Can you work these out from the model? Positions are in its coordinate system, mm. Face numbers are marked on the shaded views. A direction names the side the tool comes from. Give positions to 0.01 mm unless a question says otherwise; leave off trailing zeros. Loops run counter-clockwise (first coordinate to the right, second up) from the corner with the lowest first, then second, coordinate; pieces in that order, holes last. Notation, with made-up numbers: (19, 50.25) -> (77, 50.25) arc R11 cw to (77, 68.25) -> close; hole circle Ø10 at (4, 67.5). An arc over 180 degrees is marked (long way). Return JSON: item names as keys, results as strings. Group by question number.
Q1. Suppose I cut it at A-A, the plane z = 52. Please give me the cut outline in (x, y), and give its area (3 significant figures).
Q2. I need wall thicknesses on line 1 along X through (y, z) = (4.5, 71.5); line 2 along Z through (x, y) = (110, 6); line 3 along Z through (x, y) = (199.51, -9.5). Which ranges of each line are inside material? Lowest first, please. Write a range as [from, to].
Q3. Suppose I cut it at C-C, the plane y = 15.5. Count the separate pieces of the cut face and the enclosed holes in it, and give its area (3 significant figures).
Q4. Which directions (+Z, -Z, +X, -X, +Y, -Y) give clear straight access to the entire face, cutting with the end or side of a thin tool? Please do the marked faces 5, 6 and 7.
Q5. Thinking about a two-plate mould opening in Z: for the marked faces 1, 2, 3 and 4, which applies, pulls with the +Z half, pulls with the -Z half, needs draft (parallel to the pull), parting line crosses it, or undercut?
Q6. Will these pins go through, and if not, where does the flat tip stop? pin 1 (2 mm diameter, centred on y = -9, z = 119, fed in from -X); pin 2 (5 mm diameter, centred on x = 99.5, y = 15.5, fed in from +Z); pin 3 (6 mm diameter, centred on x = 110.5, z = 111.5, fed in from -Y).
Q7. Suppose I cut it at B-B, the plane x = 156. Please give me the cut outline in (y, z).
```python
from build123d import *

# Parameters (mm, degrees)
PAD024_DEPTH    = 34.5
POCKET023_DEPTH = 31.5
SKETCH055_R     = 2.1
SKETCH055_R_2   = 2
POCKET024_DEPTH = 6.2
SKETCH057_R     = 3
SKETCH057_R_2   = 5
SKETCH057_R_3   = 3.5
PAD025_DEPTH    = 17.5
SKETCH058_R     = 2.55
SKETCH058_R_2   = 2.1
POCKET026_DEPTH = 6.2
FILLET001_R     = 3
SKETCH059_W     = 20
SKETCH059_H     = 10
POCKET027_DEPTH = 5
SKETCH060_W     = 20
SKETCH060_H     = 10
POCKET028_DEPTH = 5


with BuildPart() as part:
    # Sketch052 → Pad024 (new body)
    with BuildSketch(Plane.XZ):
        with BuildLine():
            ThreePointArc((-0.5, 13.5), (2.428932, 6.428932), (9.5, 3.5))
            Line((9.5, 3.5), (192.51, 3.5))
            ThreePointArc((192.51, 3.5), (199.581068, 6.428932), (202.51, 13.5))
            Line((202.51, 13.5), (202.51, 109.54))
            ThreePointArc((202.51, 109.54), (199.581068, 116.611068), (192.51, 119.54))
            Line((192.51, 119.54), (97.391395, 119.54))
            ThreePointArc((97.391395, 119.54), (96.36955, 119.672723), (95.415517, 120.062083))
            Line((95.415517, 120.062083), (67.291034, 136.040187))
            ThreePointArc((67.291034, 136.040187), (65.859984, 136.624227), (64.327218, 136.823311))
            Line((64.327218, 136.823311), (35.377399, 136.823311))
            ThreePointArc((35.377399, 136.823311), (30.31762, 135.448776), (26.64881, 131.703038))
            Line((26.64881, 131.703038), (2.447131, 88.412394))
            ThreePointArc((2.447131, 88.412394), (0.24888, 82.945607), (-0.5, 77.101188))
            Line((-0.5, 77.101188), (-0.5, 13.5))
        make_face()
    extrude(amount=PAD024_DEPTH)

    # Sketch054 (on Face16 of Pad024) → Pocket023 (cut)
    with BuildSketch(Plane.XZ.offset(34.5)):
        with BuildLine():
            ThreePointArc((5.5, 15.5), (8.428932, 8.428932), (15.5, 5.5))
            Line((15.5, 5.5), (186.51, 5.5))
            ThreePointArc((186.51, 5.5), (193.581068, 8.428932), (196.51, 15.5))
            Line((196.51, 15.5), (196.51, 107.54))
            ThreePointArc((196.51, 107.54), (193.581068, 114.611068), (186.51, 117.54))
            Line((186.51, 117.54), (96.852925, 117.54))
            ThreePointArc((96.852925, 117.54), (95.816521, 117.676599), (94.850903, 118.077066))
            Line((94.850903, 118.077066), (67.278075, 134.017712))
            ThreePointArc((67.278075, 134.017712), (65.829649, 134.618413), (64.275043, 134.823311))
            Line((64.275043, 134.823311), (41.153265, 134.823311))
            ThreePointArc((41.153265, 134.823311), (36.151908, 133.482781), (32.491444, 129.820596))
            Line((32.491444, 129.820596), (8.601898, 88.412711))
            ThreePointArc((8.601898, 88.412711), (6.288899, 82.824921), (5.5, 76.829005))
            Line((5.5, 76.829005), (5.5, 15.5))
        make_face()
    extrude(amount=-POCKET023_DEPTH, mode=Mode.SUBTRACT)

    # Sketch055 (on Face5 of Pocket023) → Pocket024 (cut)
    with BuildSketch(Plane.XZ.offset(34.5)):
        with Locations((199.51, 21.5)):
            Circle(SKETCH055_R)
        with Locations((199.51, 101.5)):
            Circle(SKETCH055_R)
        with Locations((199.51, 41.5)):
            Circle(SKETCH055_R)
        with Locations((199.51, 81.5)):
            Circle(SKETCH055_R)
        with Locations((199.51, 61.5)):
            Circle(SKETCH055_R)
        with Locations((2.5, 25.5)):
            Circle(SKETCH055_R)
        with Locations((2.5, 45.5)):
            Circle(SKETCH055_R)
        with Locations((2.5, 65.5)):
            Circle(SKETCH055_R)
        with Locations((7.984524, 92.743621)):
            Circle(SKETCH055_R_2)
        with Locations((17.909674, 110.107129)):
            Circle(SKETCH055_R_2)
        with Locations((27.944341, 127.407576)):
            Circle(SKETCH055_R_2)
    extrude(amount=-POCKET024_DEPTH, mode=Mode.SUBTRACT)

    # Sketch057 (on Face51 of Pocket024) → Pad025 (join)
    with BuildSketch(Plane.XZ.offset(3)):
        with Locations((74.17, 12.74)):
            Circle(SKETCH057_R)
        with Locations((64.332465, 127.473311)):
            Circle(SKETCH057_R_2)
        with Locations((105.902925, 108.54)):
            Circle(SKETCH057_R)
        with Locations((145.13, 13)):
            Circle(SKETCH057_R_3)
        with Locations((188.34, 14.18)):
            Circle(SKETCH057_R_2)
        with Locations((185.61, 111.04)):
            Circle(SKETCH057_R_2)
        with Locations((14.14, 13.53)):
            Circle(SKETCH057_R_2)
    extrude(amount=PAD025_DEPTH)

    # Sketch058 (on Face63 of Pad025) → Pocket026 (cut)
    with BuildSketch(Plane.XZ.offset(20.5)):
        with Locations((64.332465, 127.473311)):
            Circle(SKETCH058_R)
        with Locations((105.902925, 108.54)):
            Circle(SKETCH058_R_2)
        with Locations((14.14, 13.53)):
            Circle(SKETCH058_R)
        with Locations((74.17, 12.74)):
            Circle(SKETCH058_R_2)
        with Locations((145.13, 13)):
            Circle(SKETCH058_R_2)
        with Locations((188.34, 14.18)):
            Circle(SKETCH058_R)
        with Locations((185.61, 111.04)):
            Circle(SKETCH058_R)
    extrude(amount=-POCKET026_DEPTH, mode=Mode.SUBTRACT)

    # Fillet001
    fillet001_edges = [part.edges().sort_by_distance(p)[0] for p in [
        (2.428932, 0, 6.428932),
        (101.005, 0, 3.5),
        (199.581068, 0, 6.428932),
        (202.51, 0, 61.52),
        (199.581068, 0, 116.611068),
        (144.950697, 0, 119.54),
        (96.36955, 0, 119.672723),
        (81.353275, 0, 128.051135),
        (65.859984, 0, 136.624227),
        (49.852308, 0, 136.823311),
        (30.31762, 0, 135.448776),
        (14.54797, 0, 110.057716),
        (0.24888, 0, 82.945607),
        (-0.5, 0, 45.300594),
    ]]
    fillet(fillet001_edges, radius=FILLET001_R)

    # Sketch059 (on Face16 of Fillet001) → Pocket027 (cut)
    with BuildSketch(Plane(origin=(0, 0, 119.54), x_dir=(-1, 0, 0), z_dir=(0, 0, 1))):
        with Locations((-107.391395, 29.5)):
            Rectangle(SKETCH059_W, SKETCH059_H)
    extrude(amount=-POCKET027_DEPTH, mode=Mode.SUBTRACT)

    # Sketch060 (on Face5 of Pocket027) → Pocket028 (cut)
    with BuildSketch(Plane(origin=(0, 0, 3.5), x_dir=(1, 0, 0), z_dir=(0, 0, -1))):
        with Locations((107.391395, 29.5)):
            Rectangle(SKETCH060_W, SKETCH060_H)
    extrude(amount=-POCKET028_DEPTH, mode=Mode.SUBTRACT)


with BuildPart() as part_1:
    # Body006 placement: moved
    add(part.part.moved(Location((0, 20.5, 0))))


solid = part_1.part
```
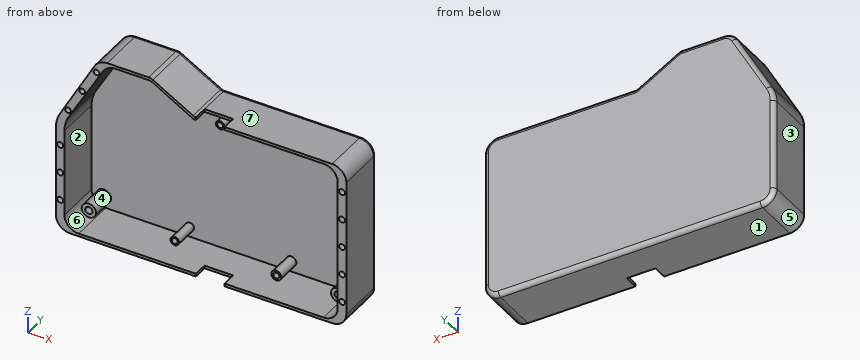
Ans:
{
 "1": {"outline": "(-0.5, -14) -> (5.5, -14) -> (5.5, 17.5) -> (196.51, 17.5) -> (196.51, -14) -> (202.51, -14) -> (202.51, 17.5) arc R3 ccw to (199.51, 20.5) -> (2.5, 20.5) arc R3 ccw to (-0.5, 17.5) -> close", "area": "983 mm^2"},
 "2": {"line 1": "x = [-0.5, 5.5], [196.51, 202.51]", "line 2": "z = [3.5, 5.5], [117.54, 119.54]", "line 3": "z = [6.36, 19.4], [23.6, 39.4], [43.6, 59.4], [63.6, 79.4], [83.6, 99.4], [103.6, 116.68]"},
 "3": {"separate pieces": "8", "enclosed holes": "1", "area": "2,640 mm^2"},
 "4": {"face 5": "-Z, -X, +Y, -Y", "face 6": "-Y", "face 7": "+Z, +X, +Y, -Y"},
 "5": {"face 1": "pulls with the -Z half", "face 2": "undercut", "face 3": "needs draft", "face 4": "undercut"},
 "6": {"pin 1": "stops at x = 18.99", "pin 2": "stops at z = 119.56", "pin 3": "stops at y = 0"},
 "7": {"outline": "(-14, 3.5) -> (17.5, 3.5) arc R3 ccw to (20.5, 6.5) -> (20.5, 116.54) arc R3 ccw to (17.5, 119.54) -> (-14, 119.54) -> (-14, 117.54) -> (17.5, 117.54) -> (17.5, 5.5) -> (-14, 5.5) -> close"}
}
